from build123d import *

# Parameters (mm, degrees)
SKETCH_1_R          = 7
EXTRUDE_1_DEPTH     = 2
CHAMFER_1_SIZE      = 1.5
SKETCH_2_R          = 1.6
CUT_EXTRUDE_1_DEPTH = 3


with BuildPart() as part:
    # Эскиз1 → Бобышка-Вытянуть1 (new body)
    with BuildSketch(Plane(origin=(0, 0, 0), x_dir=(1, 0, 0), z_dir=(0, 1, 0))):
        Circle(SKETCH_1_R)
    extrude(amount=EXTRUDE_1_DEPTH)

    # Фаска1
    chamfer_1_edges = [part.edges().sort_by_distance(p)[0] for p in [
        (-7, 2, 0),
    ]]
    chamfer(chamfer_1_edges, length=CHAMFER_1_SIZE)

    # Эскиз2 → Вырез-Вытянуть1 (cut, through all)
    with BuildSketch(Plane.XZ):
        Circle(SKETCH_2_R)
    extrude(amount=-CUT_EXTRUDE_1_DEPTH, mode=Mode.SUBTRACT)


solid = part.part
The model under review builds one solid part; all positions refer to its coordinate system, in mm. Round coordinates to 2 decimals unless told otherwise and drop trailing zeros. Loops run counter-clockwise (first coordinate to the right, second up) from the corner with the lowest first, then second, coordinate; pieces in that order, holes last. Notation, with made-up numbers: (88.25, 68.5) -> (144.25, 68.5) arc R22 cw to (144.25, 91.5) -> close; hole circle Ø9 at (-11, 49). An arc over 180 degrees is marked (long way). One line per question, with ' | ' between items. Start each with the question number.
Item 1: Add section A-A, the plane x = 0. Write out the cut boundary in (y, z), then the cut area to 4 significant figures.
Item 2: For pin 1 (2.5 mm diameter, centred on x = 0, z = 0, fed in from +Y); pin 2 (1 mm diameter, centred on x = 3.5, y = 1, fed in from -Z); pin 3 (1 mm diameter, centred on x = 1.5, y = 0.5, fed in from +Z), all flat-tipped, find the tip position at first contact; note any pin that passes through.
Item 3: Wall thickness on line 1 along Z through (x, y) = (1, 0.85); line 2 along Z through (x, y) = (-0.75, 1.75); line 3 along Z through (x, y) = (-4, 1.7): over which ranges is each line inside the solid? List them lowest first. Write a range as [from, to].
Item 4: Add section C-C, the plane y = 1.3. Write out the cut boundary in (x, z), then the cut area to 3 significant figures.
Item 5: Add section B-B, the plane z = 0. Write out the cut boundary in (x, y), then the cut area to 4 significant figures.
Return value:
1) outline: (0, -7) -> (0.5, -7) -> (2, -5.5) -> (2, -1.6) -> (0, -1.6) -> close; (0, 1.6) -> (2, 1.6) -> (2, 5.5) -> (0.5, 7) -> (0, 7) -> close | area: 19.35 mm2
2) pin 1: passes through | pin 2: stops at z = -6.13 | pin 3: stops at z = 6.93
3) line 1: z = [-6.57, -1.25], [1.25, 6.57] | line 2: z = [-5.7, -1.41], [1.41, 5.7] | line 3: z = [-4.2, 4.2]
4) outline: circle Ø12.4 at (0, 0); hole circle Ø3.2 at (0, 0) | area: 113 mm2
5) outline: (-7, 0) -> (-1.6, 0) -> (-1.6, 2) -> (-5.5, 2) -> (-7, 0.5) -> close; (1.6, 0) -> (7, 0) -> (7, 0.5) -> (5.5, 2) -> (1.6, 2) -> close | area: 19.35 mm2
